Verification items for the finished model (mm, model axes). A direction names the side the tool comes from. Round coordinates to 2 decimals unless told otherwise and drop trailing zeros. Write each loop counter-clockwise with the first axis right and the second up, starting at its lowest first coordinate (ties: lowest second). Pieces come first, ordered by that corner, then holes. Notation, with made-up numbers: M 21.25,22.5 L 55.25,22.5 A12 ccw 55.25,31.5 Z; hole C 74.25,13 d1. An arc over 180 degrees is marked long. Write each question's results on one line, items separated by ' | '.
from build123d import *

# Parameters (mm, degrees)
SKETCH1_R           = 96
BOSS_EXTRUDE1_DEPTH = 3
SKETCH1_4_R         = 97.5
SKETCH1_4_R_2       = 96
BOSS_EXTRUDE2_DEPTH = 24.22
SKETCH1_5_R         = 100
SKETCH1_5_R_2       = 97.5
BOSS_EXTRUDE3_DEPTH = 39.5


with BuildPart() as part:
    # Sketch1 → Boss-Extrude1 (new body)
    with BuildSketch(Plane(origin=(0, 0, 0), x_dir=(1, 0, 0), z_dir=(0, 1, 0))):
        with Locations(Location((0, 0, 0), (0, 0, 270))):
            Circle(SKETCH1_R)
    extrude(amount=BOSS_EXTRUDE1_DEPTH)

    # Sketch1_4 → Boss-Extrude2 (add)
    with BuildSketch(Plane(origin=(0, 0, 0), x_dir=(1, 0, 0), z_dir=(0, 1, 0))):
        with Locations(Location((0, 0, 0), (0, 0, 270))):
            Circle(SKETCH1_4_R)
        with Locations(Location((0, 0, 0), (0, 0, 270))):
            Circle(SKETCH1_4_R_2, mode=Mode.SUBTRACT)
    extrude(amount=BOSS_EXTRUDE2_DEPTH)

    # Sketch1_5 → Boss-Extrude3 (add)
    with BuildSketch(Plane(origin=(0, 0, 0), x_dir=(1, 0, 0), z_dir=(0, 1, 0))):
        with Locations(Location((0, 0, 0), (0, 0, 270))):
            Circle(SKETCH1_5_R)
        with Locations(Location((0, 0, 0), (0, 0, 270))):
            Circle(SKETCH1_5_R_2, mode=Mode.SUBTRACT)
    extrude(amount=BOSS_EXTRUDE3_DEPTH)

    # Sketch6 → Revolve1 (revolve)
    with BuildSketch(Plane(origin=(0, 3, 0), x_dir=(1, 0, 0), z_dir=(0, 0, 1))):
        Polygon((0, 0), (-13, 0), (-9, 7.918840006), (-9, 11.918840006), (-5, 14.768523744), (-4, 14.768523744), (-4, 25.768523744), (0, 25.768523744), align=None)
    revolve(axis=Axis((0, 32.411214842, 0), (0, -1, 0)))


solid = part.part
1) Sectioned sample at B-B, the plane z = 0. Record the cut outline in (x, y).
Calculated:
outline: M -100,0 L 100,0 L 100,39.5 L 97.5,39.5 L 97.5,24.22 L 96,24.22 L 96,3 L 13,3 L 9,10.92 L 9,14.92 L 5,17.77 L 4,17.77 L 4,28.77 L -4,28.77 L -4,17.77 L -5,17.77 L -9,14.92 L -9,10.92 L -13,3 L -96,3 L -96,24.22 L -97.5,24.22 L -97.5,39.5 L -100,39.5 Z
2) Draft check along Y on faces 3 (the conical face through (7.3, 10.53, 5.59)), 4 (the cylindrical face through (0.867, 23.346, 3.905)), 5 (the flat face through (1, 0, -1)). Enter one of: pulls with the +Y half, pulls with the -Y half, needs draft (parallel to the pull), parting line crosses it, or undercut.
Calculated:
face 3: pulls with the +Y half | face 4: needs draft | face 5: pulls with the -Y half
3) Sectioned sample at C-C, the plane x = 80. Record the cut outline in (y, z).
Calculated:
outline: M 0,-60 L 39.5,-60 L 39.5,-55.73 L 24.22,-55.73 L 24.22,-53.07 L 3,-53.07 L 3,53.07 L 24.22,53.07 L 24.22,55.73 L 39.5,55.73 L 39.5,60 L 0,60 Z
4) Sectioned sample at D-D, the plane z = -44.5. Record the cut outline in (x, y), and give its area (3 significant figures).
Calculated:
outline: M -89.55,0 L 89.55,0 L 89.55,39.5 L 86.75,39.5 L 86.75,24.22 L 85.06,24.22 L 85.06,3 L -85.06,3 L -85.06,24.22 L -86.75,24.22 L -86.75,39.5 L -89.55,39.5 Z | area: 813 mm²
5) Material ranges on line 1 (X direction, y = 12, z = 0); line 2 (X direction, y = 14, z = 6.5); line 3 (Z direction, x = 5.5, y = 5.5), recorded low to high. Write a range as [from, to].
Calculated:
line 1: x = [-100, -96], [-9, 9], [96, 100] | line 2: x = [-99.79, -95.78], [-6.22, 6.22], [95.78, 99.79] | line 3: z = [-99.85, -95.84], [-10.37, 10.37], [95.84, 99.85]
6) Access from +Z, -Z, +X, -X, +Y, -Y to the whole of each face (thin tool, end or side, straight path). Record for faces 1 (the flat face through (-22, 39.5, 96)), 2 (the cylindrical face through (1.172, 12.947, -8.923)).
Calculated:
face 1: +Z, -Z, +X, -X, +Y | face 2: +Y
7) Depth check by flat-ended pin: P1, Ø5, axis at x = 21.5, y = 6, coming from the -Z side; P2, Ø1.5, axis at y = 32.5, z = 44, coming from the -X side; P3, Ø5, axis at y = 26, z = 35, coming from the -X side. Enter the tip coordinate at first touch or a pass-through.
Calculated:
P1: stops at z = -98.18 | P2: stops at x = -90.16 | P3: stops at x = -94.57
8) Sectioned sample at A-A, the plane x = 0. Record the cut outline in (y, z).
Calculated:
outline: M 0,-100 L 39.5,-100 L 39.5,-97.5 L 24.22,-97.5 L 24.22,-96 L 3,-96 L 3,-13 L 10.92,-9 L 14.92,-9 L 17.77,-5 L 17.77,-4 L 28.77,-4 L 28.77,4 L 17.77,4 L 17.77,5 L 14.92,9 L 10.92,9 L 3,13 L 3,96 L 24.22,96 L 24.22,97.5 L 39.5,97.5 L 39.5,100 L 0,100 Z
